Can you work these out from the model? Positions are in its coordinate system, mm. Round coordinates to 2 decimals unless told otherwise and drop trailing zeros. Loops run counter-clockwise (first coordinate to the right, second up) from the corner with the lowest first, then second, coordinate; pieces in that order, holes last. Notation, with made-up numbers: M 48.5,36 L 64.5,36 A23 cw 64.5,56 Z; hole C 4,64 d6. An arc over 180 degrees is marked long. Answer as CSV lines item,"result".
from build123d import *

# Parameters (mm, degrees)
BOSS_EXTRUDE1_DEPTH = 4
CUT_EXTRUDE1_REACH  = 21.572
SKETCH3_R           = 1
CUT_EXTRUDE2_REACH  = 20.841
SKETCH5_R           = 1


with BuildPart() as part:
    # Sketch2 → Boss-Extrude1 (new body)
    with BuildSketch(Plane(origin=(0, 0, 0), x_dir=(1, 0, 0), z_dir=(0, 1, 0))):
        with BuildLine():
            Line((-1.955885444, -6.198750852), (-1.966664332, -5.136363636))
            ThreePointArc((-1.966664332, -5.136363636), (-1.423504748, 5.312592045), (4.27136309, -3.464889226))
            Line((4.27136309, -3.464889226), (4.800851018, -4.381989218))
            ThreePointArc((4.800851018, -4.381989218), (-1.687783454, 6.277052414), (-1.955885444, -6.198750852))
        make_face()
        with BuildLine():
            Line((0, -6.5), (0, -5.5))
            ThreePointArc((0, -5.5), (-1, -5.408326913), (-1.966664332, -5.136363636))
            Line((-1.966664332, -5.136363636), (-1.955885444, -6.198750852))
            ThreePointArc((-1.955885444, -6.198750852), (-0.989474472, -6.42424628), (0, -6.5))
        make_face()
        with BuildLine():
            ThreePointArc((4.27136309, -3.464889226), (3.57018886, -4.183748499), (2.75, -4.763139721))
            Line((2.75, -4.763139721), (3.25, -5.629165125))
            ThreePointArc((3.25, -5.629165125), (4.073439881, -5.065282572), (4.800851018, -4.381989218))
            Line((4.800851018, -4.381989218), (4.27136309, -3.464889226))
        make_face()
        with BuildLine():
            ThreePointArc((4.800851018, -4.381989218), (4.073439881, -5.065282572), (3.25, -5.629165125))
            Line((3.25, -5.629165125), (7.75, -13.423393759))
            Line((7.75, -13.423393759), (9.27136309, -12.125143264))
            Line((9.27136309, -12.125143264), (4.800851018, -4.381989218))
        make_face()
        with BuildLine():
            Line((0.101453905, -15.499485342), (0, -5.5))
            Line((0, -5.5), (0, -6.5))
            ThreePointArc((0, -6.5), (-0.989474472, -6.42424628), (-1.955885444, -6.198750852))
            Line((-1.955885444, -6.198750852), (-1.865210427, -15.135848978))
            Line((-1.865210427, -15.135848978), (0.101453905, -15.499485342))
        make_face()
    extrude(amount=BOSS_EXTRUDE1_DEPTH)

    # Sketch3 → Cut-Extrude1 (cut, up to next)
    with BuildSketch(Plane(origin=(-2.018569638, 0, 0.020480231), x_dir=(0.010145390476883202, 0, 0.9999485342016716), z_dir=(-0.9999485342016717, 0, 0.010145390476883204)), mode=Mode.PRIVATE) as cut_extrude1_sk1:
        with Locations((12.116146712, 2)):
            Circle(SKETCH3_R)
    cut_extrude1_tool1 = extrude(cut_extrude1_sk1.sketch, amount=-CUT_EXTRUDE1_REACH, mode=Mode.PRIVATE) & part.part
    add(cut_extrude1_tool1.solids().sort_by_distance((-1.895647, 2, 12.136003))[0], mode=Mode.SUBTRACT)

    # Sketch5 → Cut-Extrude2 (cut, up to next)
    with BuildSketch(Plane(origin=(1.703181272, 0, -0.983332166), x_dir=(-0.5000000000000019, 0, -0.8660254037844377), z_dir=(0.8660254037844377, 0, -0.5000000000000019)), mode=Mode.PRIVATE) as cut_extrude2_sk1:
        with Locations((-12.136363636, 2)):
            Circle(SKETCH5_R)
    cut_extrude2_tool1 = extrude(cut_extrude2_sk1.sketch, amount=-CUT_EXTRUDE2_REACH, mode=Mode.PRIVATE) & part.part
    add(cut_extrude2_tool1.solids().sort_by_distance((7.771363, 2, 9.527067))[0], mode=Mode.SUBTRACT)


solid = part.part
Item 1: If we section it at C-C on z = 7.5: Write out the boundary of the cut face in (x, y).
Output:
outline,"M -1.94,0 L 0.02,0 L 0.02,4 L -1.94,4 Z; M 4.33,0 L 6.6,0 L 6.6,4 L 4.33,4 Z"
Item 2: If I drill on line 1 along X through (y, z) = (1.95, 0); line 2 along Z through (x, y) = (3, 2.65); line 3 along Z through (x, y) = (5, 1.25), over which ranges is the centre line in solid material (lowest first)? Write a range as from..to.
Output:
line 1,"x = -6.5..-5.5, 5.5..6.5"
line 2,"z = -5.77..-4.61, 4.61..5.2"
line 3,"z = -4.15..-2.29, 2.29..4.15, 4.73..8.66"
Item 3: If we section it at B-B on y = 3.25: Write out the boundary of the cut face in (x, z), then the cut area to 3 significant figures.
Output:
outline,"M -1.96,6.2 A6.5 ccw long 4.8,4.38 L 9.27,12.13 L 7.75,13.42 L 2.75,4.76 A5.5 cw long 0,5.5 L 0.1,15.5 L -1.87,15.14 Z"
area,"69.6 mm2"
Item 4: We'd pull the mould along Z, two halves only. Please class faces 1 (the face through (7.07, 1.97, 8.31)), 2 (the face through (-0.4, 0, 6.1)), 3 (the face through (8.5, 1.972, 12.783)), 4 (the face through (6.47, 1.62, 9.21)): released by +Z, released by -Z, zero draft, split by the parting line, or undercut.
Output:
face 1,"undercut"
face 2,"zero draft"
face 3,"released by +Z"
face 4,"undercut"
Item 5: If we section it at A-A on z = 0: Write out the boundary of the cut face in (x, y), then the cut area to 3 significant figures.
Output:
outline,"M -6.5,0 L -5.5,0 L -5.5,4 L -6.5,4 Z; M 5.5,0 L 6.5,0 L 6.5,4 L 5.5,4 Z"
area,"8.00 mm2"
Item 6: If we section it at D-D on x = -0.5: State how many separate pieces and enclosed holes the cut face has, then the cut area to 3 significant figures.
Output:
separate pieces,"2"
enclosed holes,"1"
area,"40.5 mm2"
